```python
from build123d import *

# Parameters (mm, degrees)
BOSS_EXTRUDE1_DEPTH = 20
LOFT1_START         = -34.8
LOFT1_DEPTH         = 69.6
LOFT1_START_2       = -28
LOFT1_2_DEPTH       = 56
BOSS_EXTRUDE2_START = -2
BOSS_EXTRUDE2_DEPTH = 50
BOSS_EXTRUDE3_DEPTH = 2.3
BOSS_EXTRUDE4_DEPTH = 2.3
SKETCH9_W           = 56.929943861
SKETCH9_H           = 73.17042397
BOSS_EXTRUDE5_DEPTH = 34
SKETCH10_W          = 54
SKETCH10_H          = 69.6
SKETCH10_W_2        = 50
SKETCH10_H_2        = 65.6
BOSS_EXTRUDE6_DEPTH = 10
SKETCH11_W          = 50
SKETCH11_H          = 65.6
SKETCH11_W_2        = 49
SKETCH11_H_2        = 64.6
BOSS_EXTRUDE7_DEPTH = 30
CUT_EXTRUDE1_START  = -69.6
SKETCH7_R           = 5.3
CUT_EXTRUDE1_DEPTH  = 2.5
CUT_EXTRUDE2_DEPTH  = 70


with BuildPart() as part:
    # Sketch1 → Boss-Extrude1 (new body)
    with BuildSketch(Plane(origin=(0, 0, 0), x_dir=(1, 0, 0), z_dir=(0, 1, 0))):
        Polygon((27, 34.8), (-27, 34.8), (-27, 0), (-27, -34.8), (27, -34.8), (27, 0), align=None)
        Polygon((25, 0), (25, 32.8), (-25, 32.8), (-25, 0), (-25, -32.8), (25, -32.8), align=None, mode=Mode.SUBTRACT)
    extrude(amount=BOSS_EXTRUDE1_DEPTH)

    # Loft1: read off the stored shape, not the designer's step
    # Loft1 outline → Loft1 (add)
    with BuildSketch(Plane.XY.offset(LOFT1_START)):
        Polygon((-27, 20), (27, 20), (25, 35), (-25, 35), align=None)
    extrude(amount=LOFT1_DEPTH)

    # Loft1 2 outline → Loft1 2 (cut)
    with BuildSketch(Plane.YZ.offset(LOFT1_START_2)):
        Polygon((20, 34.8), (35, 32.8), (35, 34.8), align=None)
        Polygon((35, -32.8), (20, -34.8), (35, -34.8), align=None)
    extrude(amount=LOFT1_2_DEPTH, mode=Mode.SUBTRACT)

    # Cut-Loft1: read off the stored shape, not the designer's step
    # Cut-Loft1: loft between two sections, ruled curve by curve
    cut_loft1_from = [
        Edge.make_line((-25, 20, 32.8), (-25, 20, -32.8)),
        Edge.make_line((-25, 20, -32.8), (25, 20, -32.8)),
        Edge.make_line((25, 20, 32.8), (-25, 20, 32.8)),
        Edge.make_line((25, 20, -32.8), (25, 20, 32.8)),
    ]
    cut_loft1_to = [
        Edge.make_line((-23, 35, 30.8), (-23, 35, -30.8)),
        Edge.make_line((-23, 35, -30.8), (23, 35, -30.8)),
        Edge.make_line((23, 35, 30.8), (-23, 35, 30.8)),
        Edge.make_line((23, 35, -30.8), (23, 35, 30.8)),
    ]
    cut_loft1 = Solid(Shell([*[Face.make_surface_from_curves(cut_loft1_from[k], cut_loft1_to[k]) for k in range(4)], Face(Wire(cut_loft1_from)), Face(Wire(cut_loft1_to))]))
    add(cut_loft1, mode=Mode.SUBTRACT)

    # Sketch2 → Boss-Extrude2 (add)
    with BuildSketch(Plane(origin=(27, 0, 0), x_dir=(0, 0, -1), z_dir=(1, 0, 0)).offset(BOSS_EXTRUDE2_START)):
        with BuildLine():
            Line((32.8, 35), (32.8, 38.5))
            ThreePointArc((32.8, 38.5), (32.653553391, 38.853553391), (32.3, 39))
            Line((32.3, 39), (29.6, 39))
            ThreePointArc((29.6, 39), (29.246446609, 38.853553391), (29.1, 38.5))
            Line((29.1, 38.5), (29.1, 37.468550682))
            ThreePointArc((29.1, 37.468550682), (29.138060234, 37.277208966), (29.246446609, 37.114997291))
            Line((29.246446609, 37.114997291), (31.361443901, 35))
            Line((31.361443901, 35), (32.8, 35))
        make_face()
    extrude(amount=-BOSS_EXTRUDE2_DEPTH)


with BuildPart() as body_2:
    # Sketch5 → Boss-Extrude3 (new body)
    with BuildSketch(Plane.XZ):
        with BuildLine():
            Line((-25, -34.8), (-25, -9.8))
            ThreePointArc((-25, -9.8), (0, 15.2), (25, -9.8))
            Line((25, -9.8), (25, -34.8))
            Line((25, -34.8), (27, -34.8))
            Line((27, -34.8), (27, 34.8))
            Line((27, 34.8), (-27, 34.8))
            Line((-27, 34.8), (-27, -34.8))
            Line((-27, -34.8), (-25, -34.8))
        make_face()
    extrude(amount=BOSS_EXTRUDE3_DEPTH)

    # Sketch6 → Boss-Extrude4 (add)
    with BuildSketch(Plane.XZ.offset(2.3)):
        with BuildLine():
            Line((22.7, -34.8), (27, -34.8))
            Line((27, -34.8), (27, 34.8))
            Line((27, 34.8), (-27, 34.8))
            Line((-27, 34.8), (-27, -34.8))
            Line((-27, -34.8), (-22.7, -34.8))
            Line((-22.7, -34.8), (-22.7, -9.8))
            ThreePointArc((-22.7, -9.8), (0, 12.9), (22.7, -9.8))
            Line((22.7, -9.8), (22.7, -34.8))
        make_face()
    extrude(amount=BOSS_EXTRUDE4_DEPTH)


with BuildPart() as body_2_2:
    # Sketch9 → Boss-Extrude5 (new body)
    with BuildSketch(Plane(origin=(0, 20, 0), x_dir=(-1, 0, 0), z_dir=(0, 1, 0))):
        with Locations((0.264790437, -0.308922176)):
            Rectangle(SKETCH9_W, SKETCH9_H)
    extrude(amount=BOSS_EXTRUDE5_DEPTH)


with BuildPart() as part_1:
    add(part.part)

    # Combine1: cut body 2 2
    add(body_2_2.part, mode=Mode.SUBTRACT)

    # Sketch10 → Boss-Extrude6 (add)
    with BuildSketch(Plane(origin=(0, 20, 0), x_dir=(1, 0, 0), z_dir=(0, 1, 0))):
        Rectangle(SKETCH10_W, SKETCH10_H)
        Rectangle(SKETCH10_W_2, SKETCH10_H_2, mode=Mode.SUBTRACT)
    extrude(amount=BOSS_EXTRUDE6_DEPTH)

    # Sketch11 → Boss-Extrude7 (add)
    with BuildSketch(Plane(origin=(0, 30, 0), x_dir=(1, 0, 0), z_dir=(0, 1, 0))):
        Rectangle(SKETCH11_W, SKETCH11_H)
        Rectangle(SKETCH11_W_2, SKETCH11_H_2, mode=Mode.SUBTRACT)
    extrude(amount=-BOSS_EXTRUDE7_DEPTH)

    # Sketch7 → Cut-Extrude1 (cut)
    with BuildSketch(Plane.XY.offset(34.8).offset(CUT_EXTRUDE1_START)):
        with Locations((0, 10)):
            Circle(SKETCH7_R)
    extrude(amount=CUT_EXTRUDE1_DEPTH, mode=Mode.SUBTRACT)

    # Sketch8 → Cut-Extrude2 (cut)
    with BuildSketch(Plane.ZY.offset(27)):
        with BuildLine():
            Line((22.750806662, 6.15), (25.849193338, 6.15))
            ThreePointArc((25.849193338, 6.15), (26.95, 4), (25.849193338, 1.85))
            Line((25.849193338, 1.85), (22.750806662, 1.85))
            ThreePointArc((22.750806662, 1.85), (21.65, 4), (22.750806662, 6.15))
        make_face()
        with BuildLine():
            Line((-25.849193338, 6.15), (-22.750806662, 6.15))
            ThreePointArc((-22.750806662, 6.15), (-21.65, 4), (-22.750806662, 1.85))
            Line((-22.750806662, 1.85), (-25.849193338, 1.85))
            ThreePointArc((-25.849193338, 1.85), (-26.95, 4), (-25.849193338, 6.15))
        make_face()
    extrude(amount=-CUT_EXTRUDE2_DEPTH, mode=Mode.SUBTRACT)


solid = part_1.part
```
The model under review builds one solid part; all positions refer to its coordinate system, in mm. A direction names the side the tool comes from. Give positions to 0.01 mm unless a question says otherwise; leave off trailing zeros. Write each loop counter-clockwise with the first axis right and the second up, starting at its lowest first coordinate (ties: lowest second). Pieces come first, ordered by that corner, then holes.
(1) Consider section D-D, the plane y = 19.75. Give the boundary of the cut face in (x, z).
(2) Tool access review of faces 1 (the cylindrical face through (-1.149, 4.826, -33.567)), 2 (the flat face through (0, 18, -34.8)), 3 (the flat face through (-26, 30, 0)), 4 (the flat face through (0, 15, 32.3)), 5 (the flat face through (26, 6.15, -24)): name each direction out of +Z, -Z, +X, -X, +Y, -Y from which nothing blocks a thin tool from reaching the whole face with its end or side.
(3) Consider section C-C, the plane z = -10. Give the boundary of the cut face in (x, y), and give its area (3 significant figures).
(4) The part is to be moulded in two halves that separate along Y. For faces 6 (the flat face through (24.5, 15, 0)), 7 (the cylindrical face through (25.73, 3.96, -26.95)), 8 (the flat face through (-26, 0, 0)), say which applies: released by +Y, released by -Y, zero draft, split by the parting line, or undercut.
(5) To check wall thickness, follow L1, parallel to X at y = 7.25, z = -6; L2, parallel to Y at x = 0, z = -33.2; L3, parallel to Z at x = -5, y = 27.5. State the ranges of each line that lie inside material, in increasing order.
(6) Consider section B-B, the plane x = 0. Give the boundary of the cut face in (y, z).
(7) Consider section A-A, the plane x = 19. Give the boundary of the cut face in (y, z), and give its area (3 significant figures).
Returned:
1. outline: (-27, -34.8) - (27, -34.8) - (27, 34.8) - (-27, 34.8) - close; hole (-24.5, -32.3) - (24.5, -32.3) - (24.5, 32.3) - (-24.5, 32.3) - close
2. face 1: -Z
2. face 2: -Z, +X, -X, +Y, -Y
2. face 3: +Z, -Z, +X, -X, +Y
2. face 4: +Y, -Y
2. face 5: +X, -X
3. outline: (-27, 0) - (-24.5, 0) - (-24.5, 30) - (-27, 30) - close; (24.5, 0) - (27, 0) - (27, 30) - (24.5, 30) - close
3. area: 150 mm2
4. face 6: zero draft
4. face 7: undercut
4. face 8: released by -Y
5. L1: x = -27 to -24.5, 24.5 to 27
5. L2: y = 0 to 4.7, 15.3 to 30
5. L3: z = -34.8 to -32.3, 32.3 to 34.8
6. outline: (0, -34.8) - (4.7, -34.8) - (4.7, -32.3) - (0, -32.3) - close; (0, 32.3) - (30, 32.3) - (30, 34.8) - (0, 34.8) - close; (15.3, -34.8) - (30, -34.8) - (30, -32.3) - (15.3, -32.3) - close
7. outline: (0, -34.8) - (30, -34.8) - (30, -32.3) - (0, -32.3) - close; (0, 32.3) - (30, 32.3) - (30, 34.8) - (0, 34.8) - close
7. area: 150 mm2
